```python
from build123d import *

# Parameters (mm, degrees)
SKETCH1_W                = 54
SKETCH1_H                = 54
SKETCH1_W_2              = 50
SKETCH1_H_2              = 50
BOSS_EXTRUDE1_DEPTH      = 50
BOSS_EXTRUDE2_DEPTH      = 25
BOSS_EXTRUDE2_DEPTH_BACK = 125
SKETCH2_W                = 54
SKETCH2_H                = 2
SKETCH3_R                = 3
CUT_EXTRUDE1_DEPTH       = 25
SKETCH4_R                = 3
CUT_EXTRUDE2_DEPTH       = 25


with BuildPart() as part:
    # Sketch1 → Boss-Extrude1 (new, symmetric)
    with BuildSketch(Plane.XY):
        Rectangle(SKETCH1_W, SKETCH1_H)
        Rectangle(SKETCH1_W_2, SKETCH1_H_2, mode=Mode.SUBTRACT)
    extrude(amount=BOSS_EXTRUDE1_DEPTH, both=True)

    # Sketch2 → Boss-Extrude2 (add, two sides: drawn at the far end of the back side and taken through both)
    with BuildSketch(Plane.XY.offset(50).offset(-BOSS_EXTRUDE2_DEPTH_BACK)):
        with Locations((0, -26)):
            Rectangle(SKETCH2_W, SKETCH2_H)
    extrude(amount=BOSS_EXTRUDE2_DEPTH + BOSS_EXTRUDE2_DEPTH_BACK)

    # Sketch3 → Cut-Extrude1 (cut)
    with BuildSketch(Plane(origin=(0, -25, 0), x_dir=(1, 0, 0), z_dir=(0, 1, 0))):
        with Locations(Location((-10, -62.5, 0), (0, 0, 180))):
            Circle(SKETCH3_R)
        with Locations(Location((10, -62.5, 0), (0, 0, 180))):
            Circle(SKETCH3_R)
        with Locations(Location((10, 62.5, 0), (0, 0, 180))):
            Circle(SKETCH3_R)
        with Locations(Location((-10, 62.5, 0), (0, 0, 180))):
            Circle(SKETCH3_R)
    extrude(amount=-CUT_EXTRUDE1_DEPTH, mode=Mode.SUBTRACT)

    # Sketch4 → Cut-Extrude2 (cut)
    with BuildSketch(Plane(origin=(0, 27, 0), x_dir=(1, 0, 0), z_dir=(0, 1, 0))):
        with Locations(Location((15, 7.5, 0), (0, 0, 180))):
            Circle(SKETCH4_R)
        with Locations(Location((15, -7.5, 0), (0, 0, 180))):
            Circle(SKETCH4_R)
    extrude(amount=-CUT_EXTRUDE2_DEPTH, mode=Mode.SUBTRACT)


solid = part.part
```
CAD build for the part. Positions are in the model's coordinates, mm. A direction names the side the tool comes from. Round coordinates to 2 decimals unless told otherwise and drop trailing zeros. Order: outer loops, then holes, each group sorted by start corner. A loop starts at its lowest first (then second) coordinate and runs counter-clockwise, first axis right, second up.
Item 1: Tool access for faces 4 (the face through (18, 26, -7.4)), 5 (the face through (-9.609, -25.986, -59.526)), 6 (the face through (0, 26, -50)), 7 (the face through (-25, 0, 1)): list every direction of +Z, -Z, +X, -X, +Y, -Y with a clear straight run to the whole face (end or side of a thin tool).
Item 2: Probe line 1 along Z through (x, y) = (15, 25.65); line 2 along Z through (x, y) = (10, -26.4); line 3 along Y through (x, z) = (19.5, -2). List the from-to ranges inside material, lowest first.
Item 3: Saw through at B-B on z = 62.5. Write the cut outline in (x, y), then the cut area to 3 significant figures.
Item 4: Saw through at A-A on x = -23. Write the cut outline in (y, z), then the cut area to 3 significant figures.
Item 5: Saw through at D-D on x = 15. Write the cut outline in (y, z).
Item 6: Mould opens along Z. For faces 1 (the face through (18, 26, 7.6)), 2 (the face through (0, 26, 50)), 3 (the face through (0, -27, -1)) say: pulls with the +Z half, pulls with the -Z half, needs draft (parallel to the pull), parting line crosses it, or undercut.
Item 7: Saw through at C-C on y = -6. Write the cut outline in (x, z), then the cut area to 3 significant figures.
Reported:
1. face 4: +Y
1. face 5: +Y, -Y
1. face 6: -Z, +X, -X, +Y
1. face 7: +Z, -Z
2. line 1: z = -50 to -10.5, -4.5 to 4.5, 10.5 to 50
2. line 2: z = -75 to -65.5, -59.5 to 59.5, 65.5 to 75
2. line 3: y = -27 to -25, 25 to 27
3. outline: (-27, -27) - (-13, -27) - (-13, -25) - (-27, -25) - close; (-7, -27) - (7, -27) - (7, -25) - (-7, -25) - close; (13, -27) - (27, -27) - (27, -25) - (13, -25) - close
3. area: 84.0 mm2
4. outline: (-27, -75) - (-25, -75) - (-25, 75) - (-27, 75) - close; (25, -50) - (27, -50) - (27, 50) - (25, 50) - close
4. area: 500 mm2
5. outline: (-27, -75) - (-25, -75) - (-25, 75) - (-27, 75) - close; (25, -50) - (27, -50) - (27, -10.5) - (25, -10.5) - close; (25, -4.5) - (27, -4.5) - (27, 4.5) - (25, 4.5) - close; (25, 10.5) - (27, 10.5) - (27, 50) - (25, 50) - close
6. face 1: undercut
6. face 2: pulls with the +Z half
6. face 3: needs draft
7. outline: (-27, -50) - (-25, -50) - (-25, 50) - (-27, 50) - close; (25, -50) - (27, -50) - (27, 50) - (25, 50) - close
7. area: 400 mm2
